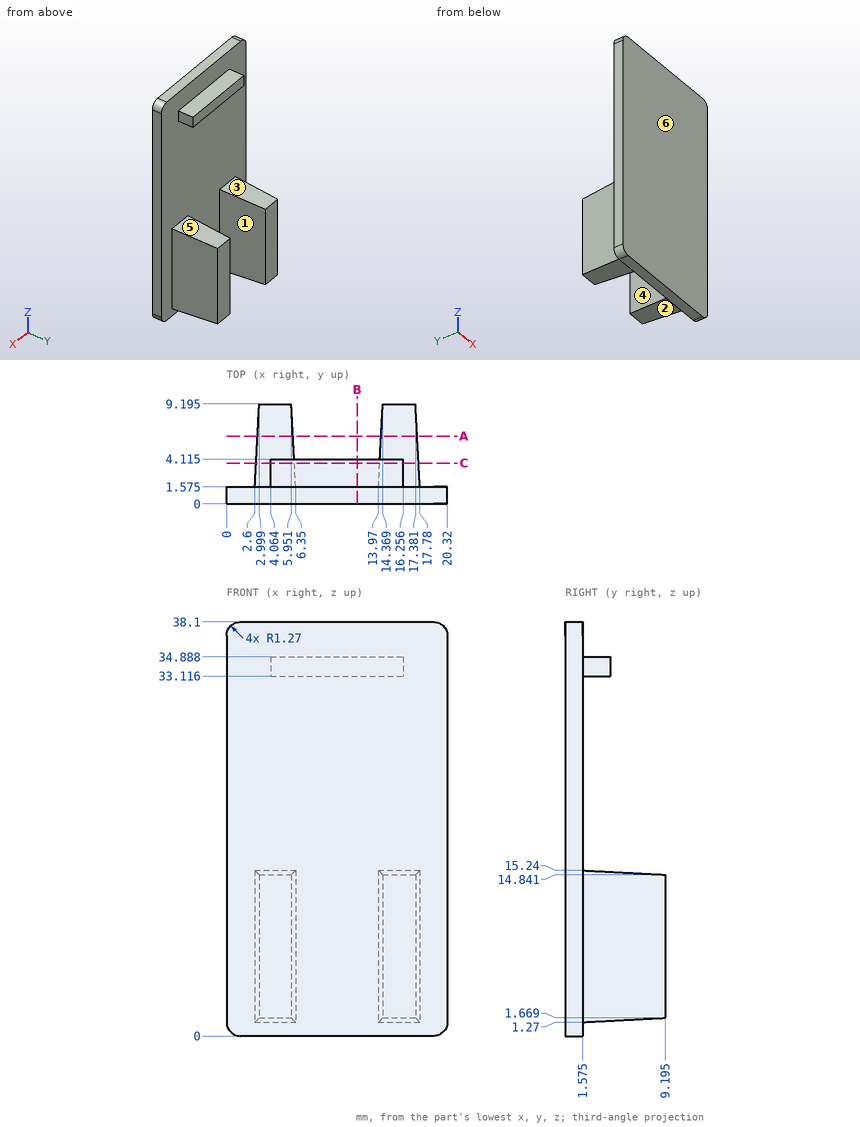
Answer from the drawing. Dimensions are ordinates in mm from the lowest x, y and z of the part. A direction names the side the tool comes from. Give positions to 0.01 mm unless a question says otherwise; leave off trailing zeros. Write each loop counter-clockwise with the first axis right and the second up, starting at its lowest first coordinate (ties: lowest second). Pieces come first, ordered by that corner, then holes. Notation, with made-up numbers: (-34, 84.5) -> (10, 84.5) arc R5 cw to (10, 92.5) -> close; hole circle Ø5 at (-4.5, 26.25). An arc over 180 degrees is marked (long way). Use a Markdown table: item, result.
(1) Flat-ended cylindrical pins translate along their axes: P1, Ø2, axis at x = 8.5, z = 4, coming from the +Y side (1 decimal); P2, Ø3, axis at x = 13, y = 2.5, coming from the -Z side; P3, Ø2, axis at x = 11.5, y = 3, coming from the +Z side; P4, Ø1.5, axis at x = 3, y = 8, coming from the -Z side. Find the tip coordinate at first contact, or state that the pin passes through.
Return value:
| item | result |
|---|---|
| P1 | y = 1.6 |
| P2 | z = 0 |
| P3 | z = 34.89 |
| P4 | z = 1.57 |
(2) Determine the mould class of the marked faces 1, 2 and 3 for opening direction Z: released by +Z, released by -Z, zero draft, split by the parting line, or undercut.
Return value:
| item | result |
|---|---|
| face 1 | zero draft |
| face 2 | released by -Z |
| face 3 | undercut |
(3) For the marked faces 4, 5 and 6, determine the directions among +Z, -Z, +X, -X, +Y, -Y from which every point of the face is accessible in a straight line to the end or side of a thin tool.
Return value:
| item | result |
|---|---|
| face 4 | -Z, +Y |
| face 5 | +X, -X, +Y |
| face 6 | +Z, -Z, +X, -X, -Y |
(4) Section B-B, the plane x = 12 is taken. Determine the outline of the cut face in (y, z) (1 decimal).
Return value:
| item | result |
|---|---|
| outline | (0, 0) -> (1.6, 0) -> (1.6, 33.1) -> (4.1, 33.1) -> (4.1, 34.9) -> (1.6, 34.9) -> (1.6, 38.1) -> (0, 38.1) -> close |
(5) Section A-A, the plane y = 6.25 is taken. Determine the outline of the cut face in (x, z) (1 decimal).
Return value:
| item | result |
|---|---|
| outline | (2.8, 1.5) -> (6.1, 1.5) -> (6.1, 15) -> (2.8, 15) -> close; (14.2, 1.5) -> (17.5, 1.5) -> (17.5, 15) -> (14.2, 15) -> close |
(6) Section C-C, the plane y = 3.75 is taken. Determine the outline of the cut face in (x, z) (1 decimal).
Return value:
| item | result |
|---|---|
| outline | (2.7, 1.4) -> (6.2, 1.4) -> (6.2, 15.1) -> (2.7, 15.1) -> close; (4.1, 33.1) -> (16.3, 33.1) -> (16.3, 34.9) -> (4.1, 34.9) -> close; (14.1, 1.4) -> (17.7, 1.4) -> (17.7, 15.1) -> (14.1, 15.1) -> close |
(7) Find the intervals of material crossed by probe 1 along Y at (x, z) = (18.5, 17.5) (1 decimal); probe 2 along Z at (x, y) = (8.75, 2.5) (1 decimal); probe 3 along X at (y, z) = (7.5, 8), in increasing order. Write a range as from..to.
Return value:
| item | result |
|---|---|
| probe 1 | 0..1.6 |
| probe 2 | 33.1..34.9 |
| probe 3 | 2.91..6.04, 14.28..17.47 |
